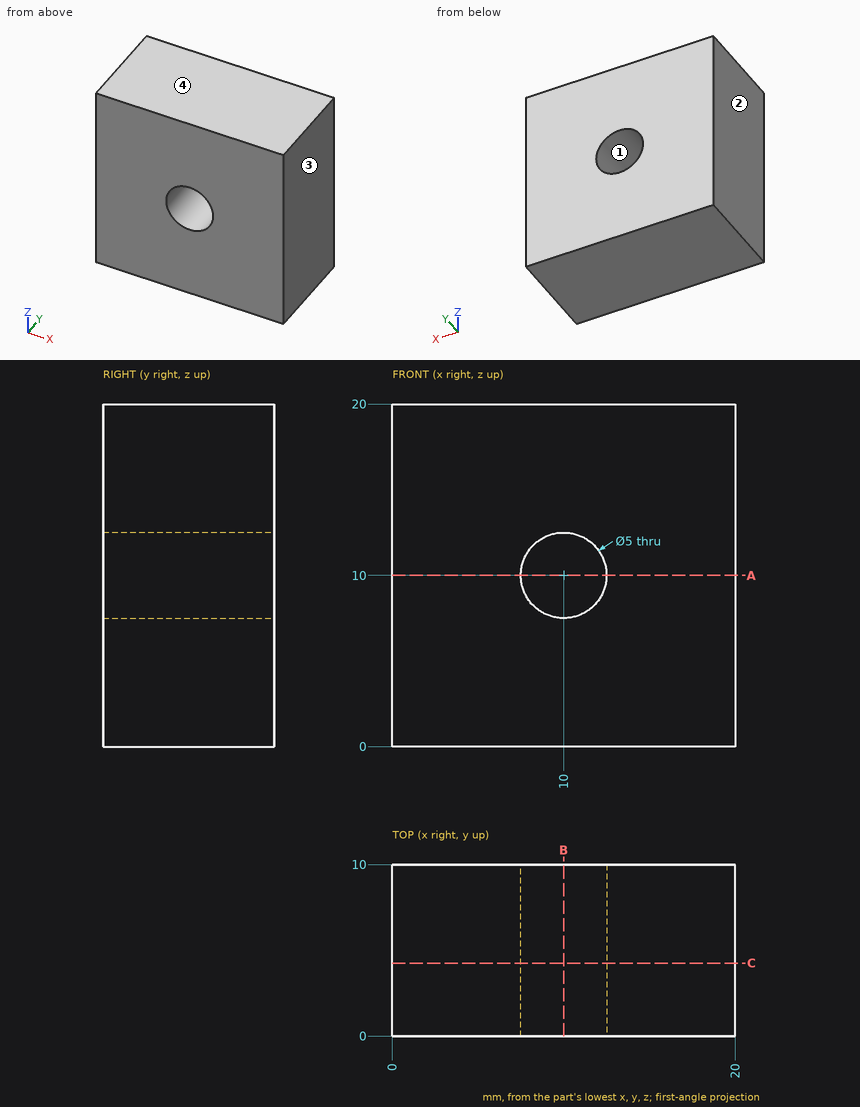
Study the drawing (mm; zero at the part's minimum x, y, z) and answer. Round coordinates to 2 decimals unless told otherwise and drop trailing zeros. Write each loop counter-clockwise with the first axis right and the second up, starting at its lowest first coordinate (ties: lowest second). Pieces come first, ordered by that corner, then holes. Notation, with made-up numbers: (71.5, 45) - (122.5, 45) arc R28 ccw to (122.5, 74) - close; hole circle Ø8 at (32, 88). An arc over 180 degrees is marked (long way). Use CSV: the item, a comma, the result in double quotes.
Q1. Find section C-C, the plane y = 4.25. Write down the section's boundary in (x, z), then the cut area to 3 significant figures.
Values:
outline,"(0, 0) - (20, 0) - (20, 20) - (0, 20) - close; hole circle Ø5 at (10, 10)"
area,"380 mm²"
Q2. Find section B-B, the plane x = 10. Write down the section's boundary in (y, z).
Values:
outline,"(0, 0) - (10, 0) - (10, 7.5) - (0, 7.5) - close; (0, 12.5) - (10, 12.5) - (10, 20) - (0, 20) - close"
Q3. Find section A-A, the plane z = 10. Write down the section's boundary in (x, y), then the cut area to 3 significant figures.
Values:
outline,"(0, 0) - (7.5, 0) - (7.5, 10) - (0, 10) - close; (12.5, 0) - (20, 0) - (20, 10) - (12.5, 10) - close"
area,"150 mm²"
Q4. Determine the mould class of the marked faces 1, 2, 3 and 4 for opening direction X: +X half, -X half, draft (parallel to the pull), parting line (faces both ways), or undercut.
Values:
face 1,"undercut"
face 2,"-X half"
face 3,"+X half"
face 4,"draft"
Q5. Straight lines are drawn through the part: line 1 along X through (y, z) = (5.5, 10); line 2 along Z through (x, y) = (7.75, 2.25). For each, find the intervals that lie inside material, in ascending order.
Values:
line 1,"x = 0 to 7.5, 12.5 to 20"
line 2,"z = 0 to 8.91, 11.09 to 20"
